Input: part model. Units: mm. Frame: model coordinates. Face numbers are marked on the shaded views. Round coordinates to 2 decimals unless told otherwise and drop trailing zeros. Loops run counter-clockwise (first coordinate to the right, second up) from the corner with the lowest first, then second, coordinate; pieces in that order, holes last. Notation, with made-up numbers: (15, -23.75) -> (55, -23.75) arc R17 cw to (55, -13.75) -> close; hole circle Ø10 at (-25, -19.75). An arc over 180 degrees is marked (long way). One line per question, with ' | ' between items. Start each with the question number.
Q1. Cut plane B-B on y = 0. Return loops of the section in (x, z) (3 decimals), and give its area (3 significant figures).
Q2. Contact query for flat-ended pins moving along their axis: P1, Ø7, axis at x = -15.5, y = 45, coming from the -Z side; P2, Ø6, axis at x = 51.5, z = -19, coming from the -Y side; P3, Ø8, axis at x = -70, z = 6, coming from the +Y side; P4, Ø6, axis at x = -76.2, y = -46.04, coming from the +Z side. Output: stop coordinate, or through.
Q3. Material intervals for L1, parallel to Y at x = -16.5, z = 10.5; L2, parallel to Y at x = -76.2, z = 26; L3, parallel to Z at x = 36, y = 41.5, sorted ascending.
Q4. Cut plane C-C on x = 76.2. Return loops of the section in (y, z).
Q5. Mould query, pull axis Y, two halves, no side actions, for the marked faces 1, 2, 3 and 4. Classes: pulls with the +Y half, pulls with the -Y half, needs draft (parallel to the pull), parting line crosses it, or undercut.
Q6. Cut plane A-A on z = -1.5. Return loops of the section in (x, y), and give its area (3 significant figures).
Q7. Cut plane D-D on x = -57.15. State how many separate pieces and enclosed holes the cut face has, and give its area (3 significant figures).
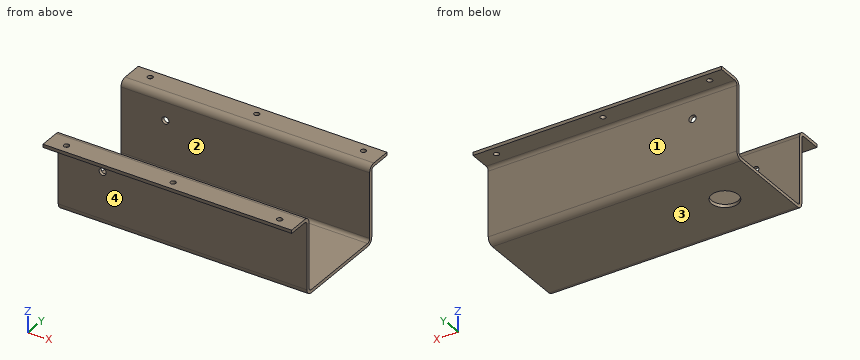
from build123d import *

# Parameters (mm, degrees)
BASE_FLANGE1_DEPTH           = 88.9
F_25_0_1495_DIAMETER_HOLE1_D = 3.7973
F_7_0_201_DIAMETER_HOLE1_D   = 5.1054
F_3_4_0_75_DIAMETER_HOLE1_D  = 19.05


# Sheet-metal steps are written as plain solids
with BuildPart() as part:
    # Sketch1 → Base-Flange1 (new, symmetric)
    with BuildSketch(Plane.YZ):
        with BuildLine():
            Line((-52.3875, 26.67), (-37.9095, 26.67))
            ThreePointArc((-37.9095, 26.67), (-34.676607796, 25.330892204), (-33.3375, 22.098))
            Line((-33.3375, 22.098), (-33.3375, -24.384))
            ThreePointArc((-33.3375, -24.384), (-32.667946102, -26.000446102), (-31.0515, -26.67))
            Line((-31.0515, -26.67), (31.0515, -26.67))
            ThreePointArc((31.0515, -26.67), (32.667946102, -26.000446102), (33.3375, -24.384))
            Line((33.3375, -24.384), (33.3375, 22.098))
            ThreePointArc((33.3375, 22.098), (34.676607796, 25.330892204), (37.9095, 26.67))
            Line((37.9095, 26.67), (52.3875, 26.67))
            Line((52.3875, 26.67), (52.3875, 24.384))
            Line((52.3875, 24.384), (37.9095, 24.384))
            ThreePointArc((37.9095, 24.384), (36.293053898, 23.714446102), (35.6235, 22.098))
            Line((35.6235, 22.098), (35.6235, -24.384))
            ThreePointArc((35.6235, -24.384), (34.284392204, -27.616892204), (31.0515, -28.956))
            Line((31.0515, -28.956), (-31.0515, -28.956))
            ThreePointArc((-31.0515, -28.956), (-34.284392204, -27.616892204), (-35.6235, -24.384))
            Line((-35.6235, -24.384), (-35.6235, 22.098))
            ThreePointArc((-35.6235, 22.098), (-36.293053898, 23.714446102), (-37.9095, 24.384))
            Line((-37.9095, 24.384), (-52.3875, 24.384))
            Line((-52.3875, 24.384), (-52.3875, 26.67))
        make_face()
    extrude(amount=BASE_FLANGE1_DEPTH, both=True)

    # #25 (0.1495) Diameter Hole1 (through all)
    with Locations(Plane.XY.offset(26.67)):
        with Locations((-76.2, 46.0375), (0, 46.0375), (76.2, 46.0375), (76.2, -46.0375), (0, -46.0375), (-76.2, -46.0375)):
            Hole(F_25_0_1495_DIAMETER_HOLE1_D / 2)

    # #7 (0.201) Diameter Hole1 (through all)
    with Locations(Plane.XZ.offset(35.6235)):
        with Locations((-57.15, 9.144)):
            Hole(F_7_0_201_DIAMETER_HOLE1_D / 2)

    # 3/4 (0.75) Diameter Hole1 (through all)
    with Locations(Plane.XY.offset(-26.67)):
        with Locations((-57.15, 0)):
            Hole(F_3_4_0_75_DIAMETER_HOLE1_D / 2)


solid = part.part
Results:
1) outline: (-88.9, -28.956) -> (-66.675, -28.956) -> (-66.675, -26.67) -> (-88.9, -26.67) -> close; (-47.625, -28.956) -> (88.9, -28.956) -> (88.9, -26.67) -> (-47.625, -26.67) -> close | area: 363 mm^2
2) P1: z = 24.38 | P2: y = -35.62 | P3: y = 35.62 | P4: z = 26.67
3) L1: -35.62 to -33.34, 33.34 to 35.62 | L2: -52.39 to -47.94, -44.14 to -35.53, 35.53 to 44.14, 47.94 to 52.39 | L3: 24.38 to 26.67
4) outline: (-52.39, 24.38) -> (-47.94, 24.38) -> (-47.94, 26.67) -> (-52.39, 26.67) -> close; (-44.14, 24.38) -> (-37.91, 24.38) arc R2.29 cw to (-35.62, 22.1) -> (-35.62, -24.38) arc R4.57 ccw to (-31.05, -28.96) -> (31.05, -28.96) arc R4.57 ccw to (35.62, -24.38) -> (35.62, 22.1) arc R2.29 cw to (37.91, 24.38) -> (44.14, 24.38) -> (44.14, 26.67) -> (37.91, 26.67) arc R4.57 ccw to (33.34, 22.1) -> (33.34, -24.38) arc R2.29 cw to (31.05, -26.67) -> (-31.05, -26.67) arc R2.29 cw to (-33.34, -24.38) -> (-33.34, 22.1) arc R4.57 ccw to (-37.91, 26.67) -> (-44.14, 26.67) -> close; (47.94, 24.38) -> (52.39, 24.38) -> (52.39, 26.67) -> (47.94, 26.67) -> close
5) face 1: pulls with the +Y half | face 2: undercut | face 3: needs draft | face 4: pulls with the -Y half
6) outline: (-88.9, -35.62) -> (88.9, -35.62) -> (88.9, -33.34) -> (-88.9, -33.34) -> close; (-88.9, 33.34) -> (88.9, 33.34) -> (88.9, 35.62) -> (-88.9, 35.62) -> close | area: 813 mm^2
7) separate pieces: 4 | enclosed holes: 0 | area: 403 mm^2
